```python
from build123d import *

# Parameters (mm, degrees)
SKETCH1_W                  = 40
SKETCH1_H                  = 25
BOSS_EXTRUDE1_DEPTH        = 2
SKETCH2_W                  = 5
SKETCH2_H                  = 20
BOSS_EXTRUDE2_DEPTH        = 10
SKETCH4_W                  = 19.965035534
SKETCH4_H                  = 6
BOSS_EXTRUDE3_DEPTH        = 5
SKETCH5_R                  = 1
CUT_EXTRUDE2_DEPTH         = 5
SKETCH6_W                  = 4
SKETCH6_H                  = 5
BOSS_EXTRUDE4_DEPTH        = 10
SKETCH8_W                  = 5
SKETCH8_H                  = 4
BOSS_EXTRUDE5_DEPTH        = 10
SKETCH9_W                  = 4
SKETCH9_H                  = 5
BOSS_EXTRUDE6_DEPTH        = 45
SKETCH12_W                 = 18
SKETCH12_H                 = 4
BOSS_EXTRUDE8_DEPTH        = 4
SKETCH13_W                 = 5
SKETCH13_H                 = 4
BOSS_EXTRUDE9_DEPTH        = 26
SKETCH14_W                 = 18
SKETCH14_H                 = 4
BOSS_EXTRUDE10_DEPTH       = 6
SKETCH16_W                 = 5.988277512
SKETCH16_H                 = 18
BOSS_EXTRUDE11_DEPTH       = 5
SKETCH15_R                 = 1
CUT_EXTRUDE3_DEPTH         = 6
SKETCH17_R                 = 3
CUT_EXTRUDE5_DEPTH         = 6
SKETCH24_R                 = 3
BOSS_EXTRUDE18_DEPTH       = 4
SKETCH24_4_R               = 3
BOSS_EXTRUDE19_DEPTH       = 6
BOSS_EXTRUDE20_START       = -1
SKETCH20_R                 = 5
SKETCH20_R_2               = 3
BOSS_EXTRUDE20_DEPTH       = 1
BOSS_EXTRUDE21_OUTLINE_R   = 2.998308623
BOSS_EXTRUDE21_OUTLINE_R_2 = 1.5
BOSS_EXTRUDE21_DEPTH       = 1
SKETCH27_R                 = 5
SKETCH27_R_2               = 2.75
BOSS_EXTRUDE22_DEPTH       = 2
SKETCH28_R                 = 2.75
CUT_EXTRUDE10_DEPTH        = 10


# Read off the part's stored shape, not the designer's step: Boss-Extrude21
with BuildPart() as part:
    # Sketch1 → Boss-Extrude1 (new body)
    with BuildSketch(Plane(origin=(0, 0, 0), x_dir=(1, 0, 0), z_dir=(0, 1, 0))):
        Rectangle(SKETCH1_W, SKETCH1_H)
    extrude(amount=BOSS_EXTRUDE1_DEPTH)

    # Sketch2 → Boss-Extrude2 (add)
    with BuildSketch(Plane(origin=(0, 2, 0), x_dir=(1, 0, 0), z_dir=(0, 1, 0))):
        with Locations((4.5, 0)):
            Rectangle(SKETCH2_W, SKETCH2_H)
    extrude(amount=BOSS_EXTRUDE2_DEPTH)

    # Sketch4 → Boss-Extrude3 (add)
    with BuildSketch(Plane(origin=(7, 0, 0), x_dir=(0, 0, -1), z_dir=(1, 0, 0))):
        with Locations((-0.017482233, 9)):
            Rectangle(SKETCH4_W, SKETCH4_H)
    extrude(amount=-BOSS_EXTRUDE3_DEPTH)

    # Sketch5 → Cut-Extrude2 (cut)
    with BuildSketch(Plane(origin=(7, 0, 0), x_dir=(0, 0, -1), z_dir=(1, 0, 0))):
        with Locations((5, 7.5)):
            Circle(SKETCH5_R)
        with Locations((-5, 7.5)):
            Circle(SKETCH5_R)
    extrude(amount=-CUT_EXTRUDE2_DEPTH, mode=Mode.SUBTRACT)

    # Sketch6 → Boss-Extrude4 (add)
    with BuildSketch(Plane(origin=(0, 2, 0), x_dir=(1, 0, 0), z_dir=(0, 1, 0))):
        with Locations((-11.527661753, -6.5)):
            Rectangle(SKETCH6_W, SKETCH6_H)
        with Locations((-11.527661753, 6.5)):
            Rectangle(SKETCH6_W, SKETCH6_H)
    extrude(amount=BOSS_EXTRUDE4_DEPTH)

    # Sketch8 → Boss-Extrude5 (add)
    with BuildSketch(Plane.ZY.offset(13.527661753)):
        with Locations((-6.5, 10)):
            Rectangle(SKETCH8_W, SKETCH8_H)
    boss_extrude5 = extrude(amount=BOSS_EXTRUDE5_DEPTH)

    # Mirror1: Boss-Extrude5 across plane
    add(boss_extrude5.mirror(Plane(origin=(0, 0, 0), x_dir=(1, 0, 0), z_dir=(0, 0, -1))))

    # Sketch9 → Boss-Extrude6 (add)
    with BuildSketch(Plane(origin=(0, 12, 0), x_dir=(1, 0, 0), z_dir=(0, 1, 0))):
        with Locations((-21.527661753, 6.5)):
            Rectangle(SKETCH9_W, SKETCH9_H)
    boss_extrude6 = extrude(amount=BOSS_EXTRUDE6_DEPTH)

    # Mirror2: Boss-Extrude5 across plane
    add(boss_extrude5.mirror(Plane(origin=(0, 0, 0), x_dir=(1, 0, 0), z_dir=(0, 0, -1))))

    # Mirror3: Boss-Extrude6 across plane
    add(boss_extrude6.mirror(Plane(origin=(0, 0, 0), x_dir=(1, 0, 0), z_dir=(0, 0, -1))))

    # Sketch12 → Boss-Extrude8 (add)
    with BuildSketch(Plane.ZY.offset(23.527661753)):
        with Locations((0, 55)):
            Rectangle(SKETCH12_W, SKETCH12_H)
        with Locations((0, 10)):
            Rectangle(SKETCH12_W, SKETCH12_H)
        with Locations((0, 32.5)):
            Rectangle(SKETCH12_W, SKETCH12_H)
    extrude(amount=-BOSS_EXTRUDE8_DEPTH)

    # Sketch13 → Boss-Extrude9 (add)
    with BuildSketch(Plane(origin=(-19.527661753, 0, 0), x_dir=(0, 0, -1), z_dir=(1, 0, 0))):
        with Locations((-6.5, 55)):
            Rectangle(SKETCH13_W, SKETCH13_H)
        with Locations((6.5, 55)):
            Rectangle(SKETCH13_W, SKETCH13_H)
    extrude(amount=BOSS_EXTRUDE9_DEPTH)

    # Sketch14 → Boss-Extrude10 (add)
    with BuildSketch(Plane(origin=(6.472338247, 0, 0), x_dir=(0, 0, -1), z_dir=(1, 0, 0))):
        with Locations((0, 55)):
            Rectangle(SKETCH14_W, SKETCH14_H)
    extrude(amount=-BOSS_EXTRUDE10_DEPTH)

    # Sketch16 → Boss-Extrude11 (add)
    with BuildSketch(Plane(origin=(0, 57, 0), x_dir=(1, 0, 0), z_dir=(0, 1, 0))):
        with Locations((3.478199491, 0)):
            Rectangle(SKETCH16_W, SKETCH16_H)
    extrude(amount=BOSS_EXTRUDE11_DEPTH)

    # Sketch15 → Cut-Extrude3 (cut)
    with BuildSketch(Plane(origin=(6.472338247, 0, 0), x_dir=(0, 0, -1), z_dir=(1, 0, 0))):
        with Locations((-5, 57.5)):
            Circle(SKETCH15_R)
        with Locations((5, 57.5)):
            Circle(SKETCH15_R)
    extrude(amount=-CUT_EXTRUDE3_DEPTH, mode=Mode.SUBTRACT)

    # Sketch17 → Cut-Extrude5 (cut)
    with BuildSketch(Plane.XZ):
        with Locations(Location((0, 0, 0), (0, 0, 270))):
            Circle(SKETCH17_R)
    extrude(amount=-CUT_EXTRUDE5_DEPTH, mode=Mode.SUBTRACT)

    # Sketch24 → Boss-Extrude18 (add)
    with BuildSketch(Plane.ZY.offset(23.527661753)):
        with Locations((0, 42)):
            Circle(SKETCH24_R)
        with BuildLine():
            Line((-4, 45), (-4, 39))
            Line((-4, 39), (0, 39))
            ThreePointArc((0, 39), (-3, 42.000000012), (2.4e-08, 45))
            Line((2.4e-08, 45), (-4, 45))
        make_face()
        with BuildLine():
            ThreePointArc((3, 42), (2.121320344, 39.878679656), (0, 39))
            Line((0, 39), (4, 39))
            Line((4, 39), (4, 45))
            Line((4, 45), (2.4e-08, 45))
            ThreePointArc((2.4e-08, 45), (2.121320352, 44.121320335), (3, 42))
        make_face()
    extrude(amount=-BOSS_EXTRUDE18_DEPTH)

    # Sketch24<4> → Boss-Extrude19 (add)
    with BuildSketch(Plane.ZY.offset(23.527661753)):
        with Locations(Location((0, 42, 0), (0, 0, 270))):
            Circle(SKETCH24_4_R)
    extrude(amount=BOSS_EXTRUDE19_DEPTH)

    # Sketch20 → Boss-Extrude20 (add)
    with BuildSketch(Plane(origin=(0, 3, 0), x_dir=(1, 0, 0), z_dir=(0, 1, 0)).offset(BOSS_EXTRUDE20_START)):
        Circle(SKETCH20_R)
        with Locations(Location((0, 0, 0), (0, 0, 90))):
            Circle(SKETCH20_R_2, mode=Mode.SUBTRACT)
    extrude(amount=BOSS_EXTRUDE20_DEPTH)

    # Boss-Extrude21 outline → Boss-Extrude21 (add)
    # profile 1 of 2: a face of its own
    with BuildSketch(Plane(origin=(0, 3, 0), x_dir=(1, 0, 0), z_dir=(0, 1, 0))):
        with BuildLine():
            ThreePointArc((2, -2.236067977), (-3, 0), (2, 2.236067977))
            Line((2, 2.236067977), (2, 4.582575695))
            ThreePointArc((2, 4.582575695), (-5, 0), (2, -4.582575695))
            Line((2, -4.582575695), (2, -2.236067977))
        make_face()
    # profile 2 of 2: a face of its own
    with BuildSketch(Plane(origin=(0, 3, 0), x_dir=(1, 0, 0), z_dir=(0, 1, 0))):
        Circle(BOSS_EXTRUDE21_OUTLINE_R)
        Circle(BOSS_EXTRUDE21_OUTLINE_R_2, mode=Mode.SUBTRACT)
    extrude(amount=BOSS_EXTRUDE21_DEPTH)

    # Sketch27 → Boss-Extrude22 (add)
    with BuildSketch(Plane(origin=(0, 4, 0), x_dir=(1, 0, 0), z_dir=(0, 1, 0))):
        Circle(SKETCH27_R)
        with Locations(Location((0, 0, 0), (0, 0, 43.341758227))):
            Circle(SKETCH27_R_2, mode=Mode.SUBTRACT)
    extrude(amount=BOSS_EXTRUDE22_DEPTH)

    # Sketch28 → Cut-Extrude10 (cut)
    with BuildSketch(Plane(origin=(0, 6, 0), x_dir=(1, 0, 0), z_dir=(0, 1, 0))):
        with Locations(Location((0, 0, 0), (0, 0, 43.341758227))):
            Circle(SKETCH28_R)
    extrude(amount=CUT_EXTRUDE10_DEPTH, mode=Mode.SUBTRACT)


solid = part.part
```
Here's how the part is built. I have some questions about the finished solid (model axes, mm). A direction names the side the tool comes from. Give positions to 0.01 mm unless a question says otherwise; leave off trailing zeros. Order: outer loops, then holes, each group sorted by start corner. A loop starts at its lowest first (then second) coordinate and runs counter-clockwise, first axis right, second up. Notation, with made-up numbers: M -29.5,89.5 L -14.5,89.5 A26 cw -14.5,103.5 Z; hole C -30.75,-27.5 d6. An arc over 180 degrees is marked long. Use a Markdown table: item, result. Add a question column.
1. Suppose I cut it at A-A (x = -18). List the corners of the cut face in (y, z) for me.
2. Suppose I cut it at B-B (y = 42). List the corners of the cut face in (x, z) for me, and give its area (3 significant figures).
3. I need wall thicknesses on probe 1 along Y at (x, z) = (4.1, 5); probe 2 along Y at (x, z) = (-18, 8); probe 3 along Z at (x, y) = (-13, 53.5). Which ranges of each line are inside material? Lowest first, please. Write a range as from..to.
4. If we mould it in two halves opening along Z, with no side actions, what happens to faces 6 (the flat face through (-22, 21, -4)), 7 (the flat face through (-22, 37, -4)), 8 (the flat face through (-20, 36, -9)), 9 (the flat face through (-3, 6, 0))? For each: +Z half, -Z half, draft (parallel to the pull), parting line (faces both ways), or undercut.
5. On a 3-axis mill with a long thin cutter (end or side, diameter ignored), from which of +Z, -Z, +X, -X, +Y, -Y can I reach the whole of each face in a straight line? I mean faces 1 (the flat face through (-9.528, 7, 7)), 2 (the flat face through (6.472, 57, 0)), 3 (the cylindrical face through (-1.5, 3.49, -0.07)), 4 (the flat face through (-13.528, 5, -6)), 5 (the flat face through (1.2, 4, 1.2)). Say none if no direction works.
6. For pin 1 Ø7 at (y, z) = (56, -1) entering from +X; pin 2 Ø6.5 at (y, z) = (8, 6.5) entering from -X; pin 3 Ø3 at (x, y) = (-21, 9) entering from +Z, each with a flat end and sliding along its axis, tell me the tip position at first contact or that it passes through.
7. Suppose I cut it at C-C (y = 23). List the corners of the cut face in (x, z) for me.
Results list:
| question | item | result |
|---|---|---|
| 1 | outline | M 0,-12.5 L 2,-12.5 L 2,12.5 L 0,12.5 Z; M 8,-9 L 12,-9 L 12,-4 L 8,-4 Z; M 8,4 L 12,4 L 12,9 L 8,9 Z; M 53,-9 L 57,-9 L 57,-4 L 53,-4 Z; M 53,4 L 57,4 L 57,9 L 53,9 Z |
| 2 | outline | M -29.53,-3 L -23.53,-3 L -23.53,-9 L -19.53,-9 L -19.53,9 L -23.53,9 L -23.53,3 L -29.53,3 Z |
| 2 | area | 108 mm² |
| 3 | probe 1 | y = 0..6.5, 8.5..12, 53..56.5, 58.5..62 |
| 3 | probe 2 | y = 0..2, 8..12, 53..57 |
| 3 | probe 3 | z = -9..-4, 4..9 |
| 4 | face 6 | undercut |
| 4 | face 7 | undercut |
| 4 | face 8 | -Z half |
| 4 | face 9 | draft |
| 5 | face 1 | +Z, -Z |
| 5 | face 2 | +Z, -Z, +X, +Y |
| 5 | face 3 | -Y |
| 5 | face 4 | +Z, -Z, -X |
| 5 | face 5 | none |
| 6 | pin 1 | stops at x = 6.47 |
| 6 | pin 2 | stops at x = -23.53 |
| 6 | pin 3 | stops at z = 9 |
| 7 | outline | M -23.53,-9 L -19.53,-9 L -19.53,-4 L -23.53,-4 Z; M -23.53,4 L -19.53,4 L -19.53,9 L -23.53,9 Z |
